Autodesk Inventor part; units mm, degrees
ref_plane "YZ Plane" through (0, 0, 0) normal (1, 0, 0) x (0, 1, 0)
ref_plane "XZ Plane" through (0, 0, 0) normal (0, 1, 0) x (-1, 0, 0)
ref_plane "XY Plane" through (0, 0, 0) normal (0, 0, 1) x (1, 0, 0)
sketch "Skizze1" plane through (0, 0, 0) normal (0, 0, 1) x (1, 0, 0)
  line L0 (-40, 29) -> (40, 29)
  line L1 (40, 29) -> (40, -29)
  line L2 (40, -29) -> (-40, -29)
  line L3 (-40, -29) -> (-40, 29)
  line L4 (-40, 29) -> (40, -29) construction
  line L5 (40, 29) -> (-40, -29) construction
  line L6 (-40, -14) -> (40, -14)
  point P0 (0, 0)
  dimension "d0" = 58
  dimension "d1" = 80
  dimension "d4" = 15
extrude "Extrusion1" add sketch "Skizze1" along normal blind 10
extrude "Extrusion2" cut sketch "Skizze1" along normal blind 5 contours L6 L1 L2 L3
sketch "Skizze2" plane through (0, 0, 0) normal (0, 0, -1) x (-1, 0, 0)
  line L0 (35, -22) -> (-35, -22) construction
  line L1 (-40, -14) -> (40, -14)
  line L2 (0, -14) -> (0, -22) construction
  line L3 (40, -14) -> (40, -29)
  line L4 (35, 25) -> (-35, 25) construction
  line L5 (-40, 29) -> (40, 29)
  point P0 (0, 0)
  point P1 (0, 25)
  dimension "d7" = 8
  dimension "d8" = 5
  dimension "d16" = 70
  dimension "d17" = 4
hole "Bohrung1" at (-35, -22, 0) at (35, -22, 0) at (-35, 25, 0) at (35, 25, 0) direction (0, 0, 1) diameter 3.4 end through all
sketch "Sketch3" plane through (0, 0, 0) normal (0, 0, -1) x (-1, 0, 0)
  line L0 (-30.5, 21) -> (-30.5, -14)
  line L1 (-4, 21) -> (-30.5, 21)
  line L2 (-4, -14) -> (-4, 21)
  line L3 (-4, -14) -> (-30.5, -14)
  point P0 (0, 0)
extrude "Extrusion3" cut sketch "Sketch3" against normal up to surface (5 mm away)
sketch "Sketch4" plane through (0, 0, 5) normal (0, 0, -1) x (-1, 0, 0)
  line L0 (-12.32, -4.25) -> (-5.72, -4.25)
  line L1 (-5.72, -4.25) -> (-5.72, 12.25)
  line L2 (-5.72, 12.25) -> (-12.32, 12.25)
  line L3 (-12.32, 12.25) -> (-12.32, -4.25)
  line L4 (-10.2773, -2.3373) -> (-7.7627, -2.3373)
  line L5 (-7.7627, 10.3373) -> (-10.2773, 10.3373)
  line L6 (-10.2773, -2.3373) -> (-7.7627, -2.3373)
  line L7 (-7.7627, -2.3373) -> (-7.7627, 10.3373)
  line L8 (-7.7627, 10.3373) -> (-10.2773, 10.3373)
  line L9 (-10.2773, 10.3373) -> (-10.2773, -2.3373)
  line L10 (-10.2773, 4) -> (-12.32, 4) construction
  line L11 (-9.02, -2.3373) -> (-9.02, -4.25) construction
  point P0 (0, 0)
  dimension "d20" = 6.6
  dimension "d21" = 16.5
extrude "Extrusion4" cut sketch "Sketch4" against normal through all contours L3 L2 L1 L0 | L9 L5 L7 L4
equation "\"d0\" = SensorBox_Width"
equation "\"d1\" = SensorBox_Length"
properties part number "Sensor_Box_Deckel" material "PBT-Kunststoff"
Work out the finished part from the listing and answer in its coordinate system (mm). A direction names the side the tool comes from. Round coordinates to 2 decimals unless told otherwise and drop trailing zeros. Loops run counter-clockwise (first coordinate to the right, second up) from the corner with the lowest first, then second, coordinate; pieces in that order, holes last. Notation, with made-up numbers: M -24,-3.5 L 15,-3.5 A9 ccw 15,11.5 Z; hole C -6,11.25 d4. An arc over 180 degrees is marked long. One line per question, with ' | ' between items. Start each with the question number.
(1) A cutting plane is placed at A-A on x = 9. Write down the section's boundary in (y, z), plus the area to 4 significant figures.
(2) A cutting plane is placed at C-C on x = -35. Write down the section's boundary in (y, z), plus the area to 3 significant figures.
(3) For a pull along X with two mould halves and no side action, classify faces 1 (the face through (1, -29, 7)), 2 (the face through (-33.5, -21.2, 7.5)), 3 (the face through (40, 0, 5)) as released by +X, released by -X, zero draft, split by the parting line, or undercut.
(4) A tool of negligible diameter and unlimited length cuts with its end or side. For faces 4 (the face through (-40, 0, 5)), 5 (the face through (35, -14, 2)), 6 (the face through (12.32, 4, 7)), 7 (the face through (4, 3, 2)), from which of +Z, -Z, +X, -X, +Y, -Y can it reach the whole face along a straight path? Write none if from no direction.
(5) Flat-ended cylindrical pins translate along their axes: pin 1 Ø2 at (x, y) = (-35, 25) entering from -Z; pin 2 Ø1.5 at (x, z) = (15, 3) entering from -Y; pin 3 Ø1.5 at (x, z) = (-25.5, 3.5) entering from -Y. Find the tip coordinate at first contact, or state that the pin passes through.
(6) Find the intervals of material crossed by line 1 (X direction, y = -22, z = 9); line 2 (Y direction, x = -35, z = 8.25); line 3 (Y direction, x = 10, z = 7), in increasing order.
(7) A cutting plane is placed at D-D on z = 3.75. Write down the section's boundary in (x, y), plus the area to 3 significant figures.
(8) A cutting plane is placed at B-B on y = -22. Write down the section's boundary in (x, z).
Geometry check:
1) outline: M -29,5 L -4.25,5 L -4.25,10 L -29,10 Z; M 12.25,5 L 21,5 L 21,0 L 29,0 L 29,10 L 12.25,10 Z | area: 247.5 mm²
2) outline: M -29,5 L -23.7,5 L -23.7,10 L -29,10 Z; M -20.3,5 L -14,5 L -14,0 L 23.3,0 L 23.3,10 L -20.3,10 Z; M 26.7,0 L 29,0 L 29,10 L 26.7,10 Z | area: 454 mm²
3) face 1: zero draft | face 2: undercut | face 3: released by +X
4) face 4: +Z, -Z, -X, +Y, -Y | face 5: -Z, +X, -X, -Y | face 6: +Z, -Z | face 7: -Z, -Y
5) pin 1: passes through | pin 2: stops at y = 21 | pin 3: stops at y = -14
6) line 1: x = -40 to -36.7, -33.3 to 33.3, 36.7 to 40 | line 2: y = -29 to -23.7, -20.3 to 23.3, 26.7 to 29 | line 3: y = -29 to -4.25, 12.25 to 29
7) outline: M -40,-14 L 4,-14 L 4,21 L 30.5,21 L 30.5,-14 L 40,-14 L 40,29 L -40,29 Z; hole C -35,25 d3.4; hole C 35,25 d3.4 | area: 2,490 mm²
8) outline: M -40,5 L -36.7,5 L -36.7,10 L -40,10 Z; M -33.3,5 L 33.3,5 L 33.3,10 L -33.3,10 Z; M 36.7,5 L 40,5 L 40,10 L 36.7,10 Z
